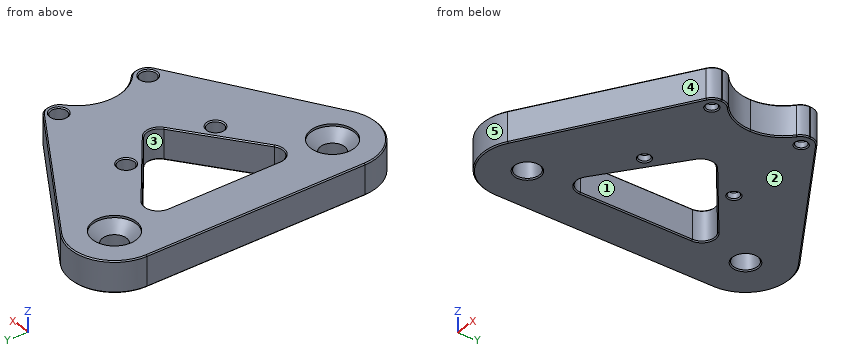
```python
from build123d import *

# Parameters (mm, degrees)
SKETCH1_R                                      = 2.75
SKETCH1_R_2                                    = 1.25
BOSS_EXTRUDE1_DEPTH                            = 7.1
SKETCH2_R                                      = 1.85
CUT_EXTRUDE1_DEPTH                             = 5.6
FILLET1_R                                      = 2.9
CSK_FOR_M5_FLAT_HEAD_MACHINE_SCREW1_AT_2_COUNT = 2
CSK_FOR_M5_FLAT_HEAD_MACHINE_SCREW1_AT_2_PITCH = 50
CUT_EXTRUDE2_REACH                             = 57.666
FILLET2_R                                      = 2.9
CHAMFER1_SIZE                                  = 0.25


with BuildPart() as part:
    # Sketch1 → Boss-Extrude1 (new body)
    with BuildSketch(Plane.XY.offset(1.1)):
        with BuildLine():
            Line((5.73970382, 12.707187863), (-27.389452344, 33.473061595))
            ThreePointArc((-27.389452344, 33.473061595), (-37.542479112, 33.749585035), (-42.7005, 25))
            Line((-42.7005, 25), (-42.7005, -25))
            ThreePointArc((-42.7005, -25), (-37.542479112, -33.749585035), (-27.389452344, -33.473061595))
            Line((-27.389452344, -33.473061595), (5.73970382, -12.707187863))
            ThreePointArc((5.73970382, -12.707187863), (6.73687966, -11.654173942), (7.0995, -10.25))
            Line((7.0995, -10.25), (7.0995, -8.535221145))
            ThreePointArc((7.0995, -8.535221145), (3.652184023, -4.871857962), (2.3995, 0))
            ThreePointArc((2.3995, 0), (3.652184023, 4.871857962), (7.0995, 8.535221145))
            Line((7.0995, 8.535221145), (7.0995, 10.25))
            ThreePointArc((7.0995, 10.25), (6.73687966, 11.654173942), (5.73970382, 12.707187863))
        make_face()
        with Locations((-32.7005, -25)):
            Circle(SKETCH1_R, mode=Mode.SUBTRACT)
        with Locations((-16.5005, -10.25)):
            Circle(SKETCH1_R_2, mode=Mode.SUBTRACT)
        with Locations((4.1995, -10.25)):
            Circle(SKETCH1_R_2, mode=Mode.SUBTRACT)
        with Locations((-32.7005, 25)):
            Circle(SKETCH1_R, mode=Mode.SUBTRACT)
        with Locations((4.1995, 10.25)):
            Circle(SKETCH1_R_2, mode=Mode.SUBTRACT)
        with Locations((-16.5005, 10.25)):
            Circle(SKETCH1_R_2, mode=Mode.SUBTRACT)
    extrude(amount=BOSS_EXTRUDE1_DEPTH)

    # Sketch2 → Cut-Extrude1 (cut)
    with BuildSketch(Plane.XY.offset(8.2)):
        with Locations((-16.5005, 10.25)):
            Circle(SKETCH2_R)
        with Locations((4.1995, 10.25)):
            Circle(SKETCH2_R)
        with Locations((-16.5005, -10.25)):
            Circle(SKETCH2_R)
        with Locations((4.1995, -10.25)):
            Circle(SKETCH2_R)
    extrude(amount=-CUT_EXTRUDE1_DEPTH, mode=Mode.SUBTRACT)

    # Fillet1
    fillet1_edges = [part.edges().sort_by_distance(p)[0] for p in [
        (7.0995, 8.535221145, 4.65),
        (7.0995, -8.535221145, 4.65),
    ]]
    fillet(fillet1_edges, radius=FILLET1_R)

    # Sketch4 → CSK for M5 Flat Head Machine Screw1 (revolve, cut)
    with BuildSketch(Plane(origin=(-32.7005, 25, 8.2), x_dir=(0, -1, 0), z_dir=(1, 0, 0))):
        Polygon((0, 0), (0, 7.1), (2.75, 7.1), (2.75, 2.75), (5, 0.5), (5, 0), align=None)
    csk_for_m5_flat_head_machine_screw1 = revolve(axis=Axis((-32.7005, 25, 14.55), (0, 0, -1)), mode=Mode.SUBTRACT)

    # CSK for M5 Flat Head Machine Screw1 at 2: CSK for M5 Flat Head Machine Screw1 ×2
    with Locations(*[(0, -i * CSK_FOR_M5_FLAT_HEAD_MACHINE_SCREW1_AT_2_PITCH, 0) for i in range(1, CSK_FOR_M5_FLAT_HEAD_MACHINE_SCREW1_AT_2_COUNT)]):
        add(csk_for_m5_flat_head_machine_screw1, mode=Mode.SUBTRACT)

    # Sketch5 → Cut-Extrude2 (cut, up to next)
    with BuildSketch(Plane.XY.offset(8.2), mode=Mode.PRIVATE) as cut_extrude2_sk1:
        Polygon((-8.232430261, 0), (-32.7005, 18.706189308), (-32.7005, -18.706189308), align=None)
    cut_extrude2_tool1 = extrude(cut_extrude2_sk1.sketch, amount=-CUT_EXTRUDE2_REACH, mode=Mode.PRIVATE) & part.part
    add(cut_extrude2_tool1.solids().sort_by_distance((-24.544477, 0, 8.2))[0], mode=Mode.SUBTRACT)

    # Fillet2
    fillet2_edges = [part.edges().sort_by_distance(p)[0] for p in [
        (-8.232430261, 0, 4.65),
        (-32.7005, -18.706189308, 4.65),
        (-32.7005, 18.706189308, 4.65),
    ]]
    fillet(fillet2_edges, radius=FILLET2_R)

    # Chamfer1
    chamfer1_edges = [part.edges().sort_by_distance(p)[0] for p in [
        (-37.542479112, -33.749585035, 8.2),
        (-19.642543112, -8.723194486, 8.2),
        (-19.642543112, -8.723194486, 1.1),
        (-32.7005, 0, 1.1),
        (-32.7005, 0, 8.2),
        (-19.642543112, 8.723194486, 1.1),
        (-19.642543112, 8.723194486, 8.2),
        (-31.08544208, -15.438480665, 8.2),
        (-31.08544208, -15.438480665, 1.1),
        (-10.107239813, 0, 8.2),
        (-10.107239813, 0, 1.1),
        (-31.08544208, 15.438480665, 8.2),
        (-31.08544208, 15.438480665, 1.1),
        (-10.824874262, -23.090124729, 8.2),
        (-35.4505, -25, 1.1),
        (-35.4505, 25, 1.1),
        (-17.7505, 10.25, 1.1),
        (2.9495, -10.25, 1.1),
        (2.9495, 10.25, 1.1),
        (6.73687966, -11.654173942, 8.2),
        (-17.7505, -10.25, 1.1),
        (-42.7005, 0, 1.1),
        (-37.542479112, 33.749585035, 1.1),
        (-10.824874262, 23.090124729, 1.1),
        (6.73687966, 11.654173942, 1.1),
        (7.0995, 10.127749244, 1.1),
        (6.73687966, -11.654173942, 1.1),
        (-10.824874262, -23.090124729, 1.1),
        (-37.542479112, -33.749585035, 1.1),
        (7.0995, 10.127749244, 8.2),
        (6.73687966, 11.654173942, 8.2),
        (-10.824874262, 23.090124729, 8.2),
        (-37.542479112, 33.749585035, 8.2),
        (-42.7005, 0, 8.2),
        (2.3495, 10.25, 8.2),
        (2.3495, 10.25, 2.6),
        (-18.3505, -10.25, 8.2),
        (-18.3505, -10.25, 2.6),
        (2.3495, -10.25, 8.2),
        (2.3495, -10.25, 2.6),
        (-18.3505, 10.25, 8.2),
        (-18.3505, 10.25, 2.6),
        (2.3995, 0, 1.1),
        (2.3995, 0, 8.2),
        (7.0995, -10.127749244, 1.1),
        (6.824329665, 8.772506505, 1.1),
        (6.824329665, -8.772506505, 1.1),
        (7.0995, -10.127749244, 8.2),
        (6.824329665, 8.772506505, 8.2),
        (6.824329665, -8.772506505, 8.2),
    ]]
    chamfer(chamfer1_edges, length=CHAMFER1_SIZE)


solid = part.part
```
Model file for the job. Use its own axes, mm. Face numbers are marked on the shaded views. A direction names the side the tool comes from. Coordinates: 2 decimals unless noted, no trailing zeros. Order: outer loops, then holes, each group sorted by start corner. A loop starts at its lowest first (then second) coordinate and runs counter-clockwise, first axis right, second up. Notation, with made-up numbers: (-16.75, -11.75) -> (33.25, -11.75) arc R23 ccw to (33.25, 21.25) -> close; hole circle Ø2 at (21.5, -27.5). An arc over 180 degrees is marked (long way). Answer as a JSON object with one key per item and string values. Group by question number.
1) Cut at B-B, the plane z = 6.5. Write the cut outline in (x, y).
2) Cut at C-C, the plane x = 4. Count the separate pieces of the cut face and the enclosed holes in it, then the cut area to 3 significant figures.
3) Pull direction X, two halves, no side cores. Call the marked faces 3, 4 and 5: +X half, -X half, draft (parallel to the pull), parting line (faces both ways), or undercut.
4) Which spindle directions (+Z, -Z, +X, -X, +Y, -Y) get a long thin tool onto all of the face, cutting with end or side? Do the marked faces 1 and 2. Say none if no direction does.
5) Flat gauge pins, fed straight in: pin 1 (1.5 mm diameter, centred on x = -16.5, y = -10.25, fed in from -Z); pin 2 (3.5 mm diameter, centred on x = 4.2, y = -10.25, fed in from +Z). Where does each tip first touch, or does it go through?
6) Drill centre lines: L1, parallel to X at y = -10.25, z = 1.7; L2, parallel to Y at x = -30.5, z = 5.75; L3, parallel to Y at x = -32, z = 7.75. Where is each one in solid material? Low to high.
7) Cut at A-A, the plane x = -23.5. Write the cut outline in (y, z), then the cut area to 3 significant figures.
Check values:
{
 "1": {"outline": "(-42.7, -25) arc R10 ccw to (-27.39, -33.47) -> (5.74, -12.71) arc R2.9 ccw to (7.1, -10.25) -> (7.1, -10.01) arc R2.9 ccw to (6.05, -7.77) arc R10.1 cw to (6.05, 7.77) arc R2.9 ccw to (7.1, 10.01) -> (7.1, 10.25) arc R2.9 ccw to (5.74, 12.71) -> (-27.39, 33.47) arc R10 ccw to (-42.7, 25) -> close; hole circle Ø7.6 at (-32.7, -25); hole circle Ø7.6 at (-32.7, 25); hole (-32.7, -12.84) arc R2.9 ccw to (-28.04, -15.14) -> (-11.25, -2.3) arc R2.9 ccw to (-11.25, 2.3) -> (-28.04, 15.14) arc R2.9 ccw to (-32.7, 12.84) -> close; hole circle Ø3.7 at (-16.5, -10.25); hole circle Ø3.7 at (-16.5, 10.25); hole circle Ø3.7 at (4.2, -10.25); hole circle Ø3.7 at (4.2, 10.25)"},
 "2": {"separate pieces": "4", "enclosed holes": "0", "area": "69.3 mm²"},
 "3": {"face 3": "undercut", "face 4": "+X half", "face 5": "parting line"},
 "4": {"face 1": "+Z, -Z", "face 2": "-Z, +X, -X, +Y, -Y"},
 "5": {"pin 1": "passes through", "pin 2": "stops at z = 2.75"},
 "6": {"L1": "x = -42.7 to -32.7, -21.64 to -17.75, -15.25 to 2.95, 5.45 to 7.1", "L2": "y = -34.75 to -27.11, -22.89 to -15.65, 15.65 to 22.89, 27.11 to 34.75", "L3": "y = -34.98 to -29.95, -20.05 to -14.73, 14.73 to 20.05, 29.95 to 34.98"},
 "7": {"outline": "(-31.04, 1.35) -> (-30.74, 1.1) -> (-11.99, 1.1) -> (-11.67, 1.35) -> (-11.67, 7.95) -> (-11.99, 8.2) -> (-30.74, 8.2) -> (-31.04, 7.95) -> close; (11.67, 1.35) -> (11.99, 1.1) -> (30.74, 1.1) -> (31.04, 1.35) -> (31.04, 7.95) -> (30.74, 8.2) -> (11.99, 8.2) -> (11.67, 7.95) -> close", "area": "275 mm²"}
}
